```python
from build123d import *

# Parameters (mm, degrees)
F1_DEPTH = 10
F2_R     = 5
F3_R     = 0.49999


# Not quite as in the source:
# - a fillet or chamfer is up to 0.001 mm smaller than in the source, because OpenCascade refuses the exact size


with BuildPart() as f1:
    # F0 (on Top) → F1 (new body)
    with BuildSketch(Plane.XY):
        with BuildLine():
            ThreePointArc((-2.2598988064, -3.2396538989), (-1.8270057081, 3.5020779749), (3.95, 0))
            ThreePointArc((3.95, 0), (4.0500202922, 1.2001209016), (4.3473214286, 2.3671283017))
            ThreePointArc((4.3473214286, 2.3671283017), (-2.9159046624, 4), (-3.5838223047, -3.4144864458))
            Line((-3.5838223047, -3.4144864458), (-2.2598988064, -3.2396538989))
        make_face()
        with BuildLine():
            ThreePointArc((4.3473214286, 2.3671283017), (4.0500202922, 1.2001209016), (3.95, 0))
            ThreePointArc((3.95, 0), (4.0500202922, -1.2001209016), (4.3473214286, -2.3671283017))
            ThreePointArc((4.3473214286, -2.3671283017), (4.7969647211, -1.2213228338), (4.95, 0))
            ThreePointArc((4.95, 0), (4.7969647211, 1.2213228338), (4.3473214286, 2.3671283017))
        make_face()
        with BuildLine():
            ThreePointArc((4.3473214286, -2.3671283017), (4.0500202922, -1.2001209016), (3.95, 0))
            ThreePointArc((3.95, 0), (3.7111266365, -1.352789373), (3.0233979302, -2.5419608485))
            Line((3.0233979302, -2.5419608485), (4.3473214286, -2.3671283017))
        make_face()
        with BuildLine():
            ThreePointArc((4.95, 0), (4.7969647211, -1.2213228338), (4.3473214286, -2.3671283017))
            Line((4.3473214286, -2.3671283017), (5.5605645672, -2.6943028782))
            ThreePointArc((5.5605645672, -2.6943028782), (5.1045520487, -1.3813088983), (4.95, 0))
        make_face()
        with BuildLine():
            ThreePointArc((18.45, 0), (12.4001209016, 7.1499797078), (4.3473214286, 2.3671283017))
            ThreePointArc((4.3473214286, 2.3671283017), (4.7969647211, 1.2213228338), (4.95, 0))
            ThreePointArc((4.95, 0), (11.2, 6.25), (17.45, 0))
            ThreePointArc((17.45, 0), (16.7255629222, -2.9207284011), (14.7201905943, -5.1643739388))
            Line((14.7201905943, -5.1643739388), (15.9334337329, -5.4915485153))
            ThreePointArc((15.9334337329, -5.4915485153), (17.790898822, -3.0203563893), (18.45, 0))
        make_face()
    extrude(amount=F1_DEPTH)

    # F2
    f2_edges = [f1.edges().sort_by_distance(p)[0] for p in [
        (4.347321, 2.367128, 5),
    ]]
    fillet(f2_edges, radius=F2_R)

    # F3 (radius 0.5 in the source; OpenCascade refuses exactly that, so slightly less here)
    f3_edges = [f1.edges().sort_by_distance(p)[0] for p in [
        (-2.259899, -3.239654, 5),
        (3.023398, -2.541961, 5),
        (5.560565, -2.694303, 5),
        (14.720191, -5.164374, 5),
        (-3.583822, -3.414486, 5),
    ]]
    fillet(f3_edges, radius=F3_R)


solid = f1.part
```
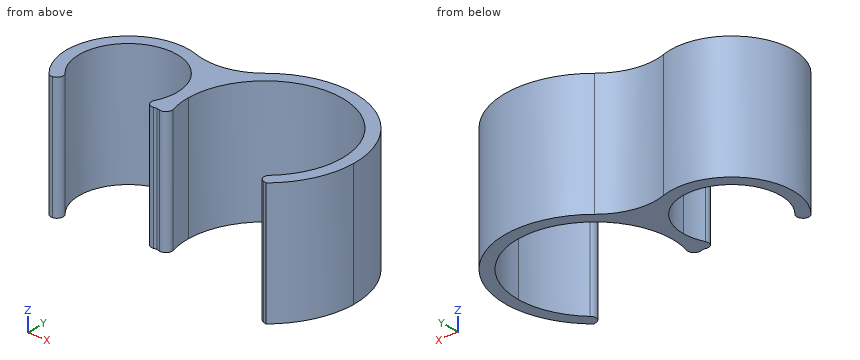
Design review of the part built by this model. Coordinates are the model's own, in mm. Give positions to 0.01 mm unless a question says otherwise; leave off trailing zeros. Order: outer loops, then holes, each group sorted by start corner. A loop starts at its lowest first (then second) coordinate and runs counter-clockwise, first axis right, second up. Notation, with made-up numbers: M 56.5,35 L 84.5,35 A13 ccw 84.5,54 Z; hole C 25.5,51.5 d5. An arc over 180 degrees is marked long. One line per question, with ' | ' between items. Start each with the question number.
Q1. We need section A-A (y = 3). Write out the cut boundary in (x, z), plus the area to 3 significant figures.
Q2. We need section B-B (x = 0). Write out the cut boundary in (y, z).
Q3. For L1, parallel to X at y = 3, z = 2.75; L2, parallel to X at y = -2, z = 7.25; L3, parallel to X at y = 5.75, z = 3.75, list the stretches that pass through material, from the lowest coordinate up. Write a range as [from, to].
Q4. We need section C-C (x = 9.25). Write out the cut boundary in (y, z).
Returned:
1) outline: M -3.94,0 L -2.57,0 L -2.57,10 L -3.94,10 Z; M 2.57,0 L 5.72,0 L 5.72,10 L 2.57,10 Z; M 16.68,0 L 17.8,0 L 17.8,10 L 16.68,10 Z | area: 56.3 mm2
2) outline: M 3.95,0 L 4.95,0 L 4.95,10 L 3.95,10 Z
3) L1: [-3.94, -2.57], [2.57, 5.72], [16.68, 17.8] | L2: [-4.53, -3.41], [3.53, 5.24], [17.12, 18.17] | L3: [6.78, 8.75], [13.65, 15.62]
4) outline: M 5.94,0 L 6.98,0 L 6.98,10 L 5.94,10 Z
